Autodesk Inventor part; units mm, degrees
ref_plane "YZ Plane" through (0, 0, 0) normal (1, 0, 0) x (0, 1, 0)
ref_plane "XZ Plane" through (0, 0, 0) normal (0, 1, 0) x (-1, 0, 0)
ref_plane "XY Plane" through (0, 0, 0) normal (0, 0, 1) x (1, 0, 0)
ref_plane "Work Plane1" through (-521.128, -68.463, 0) normal (0, 0, 1) x (-0.9986, 0.0523, 0)
ref_plane "Work Plane2" through (223.5893, -43.1165, -6.351) normal (0, -1, 0) x (1, 0, 0)
sketch "Sketch1" plane through (223.5893, -43.1165, -6.351) normal (0, -1, 0) x (1, 0, 0)
  line L0 (-282.6219, 6.351) -> (-282.6219, 0.001)
  line L1 (-173.8519, 0.001) -> (-282.6219, 0.001)
  line L2 (-282.6219, 6.351) -> (-173.8519, 6.351)
  line L3 (-283.1206, 28.576) -> (-366.4496, 6.351)
  line L4 (-283.1206, 3.176) -> (-376.14, 3.176) construction
  line L5 (-283.1206, -22.224) -> (-366.4496, 0.001)
  line L6 (-366.4496, 6.351) -> (-366.4496, 0.001)
  line L7 (-283.1206, 28.576) -> (-283.1206, -22.224)
  line L8 (-289.4706, 0.001) -> (-295.8206, 0.001)
  line L9 (-295.8206, 0.001) -> (-295.8206, 6.351)
  line L10 (-295.8206, 6.351) -> (-289.4706, 6.351)
  line L11 (-289.4706, 6.351) -> (-289.4706, 0.001)
  line L12 (-302.1706, 0.001) -> (-308.5206, 0.001)
  line L13 (-308.5206, 0.001) -> (-308.5206, 6.351)
  line L14 (-308.5206, 6.351) -> (-302.1706, 6.351)
  line L15 (-302.1706, 6.351) -> (-302.1706, 0.001)
  line L16 (-314.8706, 0.001) -> (-321.2206, 0.001)
  line L17 (-321.2206, 0.001) -> (-321.2206, 6.351)
  line L18 (-321.2206, 6.351) -> (-314.8706, 6.351)
  line L19 (-314.8706, 6.351) -> (-314.8706, 0.001)
  line L20 (-327.5706, 0.001) -> (-333.9206, 0.001)
  line L21 (-333.9206, 0.001) -> (-333.9206, 6.351)
  line L22 (-333.9206, 6.351) -> (-327.5706, 6.351)
  line L23 (-327.5706, 6.351) -> (-327.5706, 0.001)
  line L24 (-340.2706, 0.001) -> (-346.6206, 0.001)
  line L25 (-346.6206, 0.001) -> (-346.6206, 6.351)
  line L26 (-346.6206, 6.351) -> (-340.2706, 6.351)
  line L27 (-340.2706, 6.351) -> (-340.2706, 0.001)
  line L28 (-352.9706, 0.001) -> (-359.3206, 0.001)
  line L29 (-359.3206, 0.001) -> (-359.3206, 6.351)
  line L30 (-359.3206, 6.351) -> (-352.9706, 6.351)
  line L31 (-352.9706, 6.351) -> (-352.9706, 0.001)
  line L32 (-282.6219, 6.351) -> (-282.6219, 0.001)
  line L33 (-173.8519, 6.351) -> (-173.8519, 0.001)
  point P0 (-223.5893, 6.351)
  dimension "d17" = 12.7
extrude "Extrusion2" add sketch "Sketch1" against normal blind 6.35 contours L7 L5 L6 L3
properties part number "brace01"
For this review, take the finished solid that the model builds, in its own axes (mm). A direction names the side the tool comes from. Round coordinates to 2 decimals unless told otherwise and drop trailing zeros. Write each loop counter-clockwise with the first axis right and the second up, starting at its lowest first coordinate (ties: lowest second). Pieces come first, ordered by that corner, then holes. Notation, with made-up numbers: (62, -26) -> (120, -26) arc R15 ccw to (120, 1) -> close; hole circle Ø10 at (3, 60.25). An arc over 180 degrees is marked (long way). Use one line per item in the form item = value.
Q1. To check wall thickness, follow probe 1 along Z at (x, y) = (-70, -40.25); probe 2 along Z at (x, y) = (-79, -38.5); probe 3 along Z at (x, y) = (-98, -42). State the ranges of each line that lie inside material, in increasing order. Write a range as from..to.
Resolved:
probe_1 = -25.78..-6.35, 0..19.43
probe_2 = -23.38..-6.35, 0..17.03
probe_3 = -18.31..11.96
Q2. Machinability: for faces 4 (the flat face through (-133, -40, -6.35)), 5 (the flat face through (-59.531, -40, -3)), which of the approach directions +Z, -Z, +X, -X, +Y, -Y give a long, thin tool a straight path to every point of the face, cutting with its end or side? Answer none if there is none.
Resolved:
face_4 = +Y, -Y
face_5 = +Z, -Z, +X, +Y, -Y
Q3. Consider section D-D (x = -106). State the section outline as (y, z) points, then the cut area to 3 significant figures.
Resolved:
outline = (-43.12, -16.18) -> (-36.77, -16.18) -> (-36.77, -6.35) -> (-43.12, -6.35) -> close; (-43.12, 0) -> (-36.77, 0) -> (-36.77, 9.83) -> (-43.12, 9.83) -> close
area = 125 mm²
Q4. The part is to be moulded in two halves that separate along Z. For faces 1 (the flat face through (-100.61, -39.99, -17.62)), 2 (the flat face through (-95, -40, 0)), 3 (the flat face through (-93, -36.766, -8)), say which applies: released by +Z, released by -Z, zero draft, split by the parting line, or undercut.
Resolved:
face_1 = released by -Z
face_2 = undercut
face_3 = zero draft
Q5. Consider section B-B (y = -41). State the section outline as (x, z) points (3 decimals), then the cut area to 3 significant figures.
Resolved:
outline = (-142.86, -6.35) -> (-59.531, -28.575) -> (-59.531, 22.225) -> (-142.86, 0) -> close; hole (-135.731, -6.35) -> (-129.381, -6.35) -> (-129.381, 0) -> (-135.731, 0) -> close; hole (-123.031, -6.35) -> (-116.681, -6.35) -> (-116.681, 0) -> (-123.031, 0) -> close; hole (-110.331, -6.35) -> (-103.981, -6.35) -> (-103.981, 0) -> (-110.331, 0) -> close; hole (-97.631, -6.35) -> (-91.281, -6.35) -> (-91.281, 0) -> (-97.631, 0) -> close; hole (-84.931, -6.35) -> (-78.581, -6.35) -> (-78.581, 0) -> (-84.931, 0) -> close; hole (-72.231, -6.35) -> (-65.881, -6.35) -> (-65.881, 0) -> (-72.231, 0) -> close
area = 2,140 mm²
Q6. Clearance check with flat-ended pins moving along their axes: pin 1 Ø1 at (x, y) = (-110.5, -42.5) entering from -Z; pin 2 Ø3 at (x, y) = (-81.5, -40) entering from -Z; pin 3 Ø1.9 at (x, y) = (-120, -40) entering from -Z. State where each tip first meets the part, or that it passes through.
Resolved:
pin_1 = -15.11
pin_2 = -23.12
pin_3 = -12.7
Q7. Consider section C-C (x = -83.5). State the section outline as (y, z) points.
Resolved:
outline = (-43.12, -22.18) -> (-36.77, -22.18) -> (-36.77, -6.35) -> (-43.12, -6.35) -> close; (-43.12, 0) -> (-36.77, 0) -> (-36.77, 15.83) -> (-43.12, 15.83) -> close
Q8. Consider section A-A (z = -2.5). State the section outline as (x, y) points, then the cut area to 3 significant figures.
Resolved:
outline = (-142.86, -43.12) -> (-135.73, -43.12) -> (-135.73, -36.77) -> (-142.86, -36.77) -> close; (-129.38, -43.12) -> (-123.03, -43.12) -> (-123.03, -36.77) -> (-129.38, -36.77) -> close; (-116.68, -43.12) -> (-110.33, -43.12) -> (-110.33, -36.77) -> (-116.68, -36.77) -> close; (-103.98, -43.12) -> (-97.63, -43.12) -> (-97.63, -36.77) -> (-103.98, -36.77) -> close; (-91.28, -43.12) -> (-84.93, -43.12) -> (-84.93, -36.77) -> (-91.28, -36.77) -> close; (-78.58, -43.12) -> (-72.23, -43.12) -> (-72.23, -36.77) -> (-78.58, -36.77) -> close; (-65.88, -43.12) -> (-59.53, -43.12) -> (-59.53, -36.77) -> (-65.88, -36.77) -> close
area = 287 mm²
